```python
from build123d import *

# Parameters (mm, degrees)
SKETCH_1_W          = 30
SKETCH_1_H          = 34
EXTRUDE_1_DEPTH     = 30
HOLE_WIZARD_1_D     = 3.3
HOLE_WIZARD_1_DEPTH = 10
HOLE_WIZARD_2_D     = 3.3
HOLE_WIZARD_2_DEPTH = 10
HOLE_WIZARD_3_D     = 10.5


with BuildPart() as part:
    # 草图1 → 凸台-拉伸1 (new body)
    with BuildSketch(Plane(origin=(0, 0, 0), x_dir=(1, 0, 0), z_dir=(0, 1, 0))):
        with Locations((15, 17)):
            Rectangle(SKETCH_1_W, SKETCH_1_H)
    extrude(amount=EXTRUDE_1_DEPTH)

    # 孔1
    with Locations(Plane(origin=(30, 0, 0), x_dir=(0, 0, -1), z_dir=(1, 0, 0))):
        with Locations((5, 25), (29, 25), (5, 5), (29, 5)):
            Hole(HOLE_WIZARD_1_D / 2, depth=HOLE_WIZARD_1_DEPTH)

    # 孔2
    with Locations(Plane(origin=(0, 30, 0), x_dir=(1, 0, 0), z_dir=(0, 1, 0))):
        with Locations((7, 17), (15, 25), (23, 17), (15, 9)):
            Hole(HOLE_WIZARD_2_D / 2, depth=HOLE_WIZARD_2_DEPTH)

    # 孔3 (through all)
    with Locations(Plane(origin=(0, 30, 0), x_dir=(1, 0, 0), z_dir=(0, 1, 0))):
        with Locations((15, 17)):
            Hole(HOLE_WIZARD_3_D / 2)


solid = part.part
```
Check sheet for the modelled part. Datum: model origin and axes. Units: mm. A direction names the side the tool comes from. Round coordinates to 2 decimals unless told otherwise and drop trailing zeros. Loops run counter-clockwise (first coordinate to the right, second up) from the corner with the lowest first, then second, coordinate; pieces in that order, holes last. Notation, with made-up numbers: (82, 38) -> (89, 38) arc R30 ccw to (89, 61) -> close; hole circle Ø4 at (36.5, -35.75). An arc over 180 degrees is marked (long way). Answer in a Markdown table with one row per item.
Q1. Sectioned sample at A-A on z = -17. Enter the section's corners in (x, y), then the cut area to 3 significant figures.
Data:
| item | result |
|---|---|
| outline | (0, 0) -> (9.75, 0) -> (9.75, 30) -> (8.65, 30) -> (8.65, 20) -> (5.35, 20) -> (5.35, 30) -> (0, 30) -> close; (20.25, 0) -> (30, 0) -> (30, 30) -> (24.65, 30) -> (24.65, 20) -> (21.35, 20) -> (21.35, 30) -> (20.25, 30) -> close |
| area | 519 mm^2 |
Q2. Sectioned sample at C-C on y = 20.75. Enter the section's corners in (x, z).
Data:
| item | result |
|---|---|
| outline | (0, -34) -> (30, -34) -> (30, 0) -> (0, 0) -> close; hole circle Ø3.3 at (7, -17); hole circle Ø10.5 at (15, -17); hole circle Ø3.3 at (15, -25); hole circle Ø3.3 at (15, -9); hole circle Ø3.3 at (23, -17) |
Q3. Sectioned sample at B-B on x = 15. Enter the section's corners in (y, z), then the cut area to 3 significant figures.
Data:
| item | result |
|---|---|
| outline | (0, -34) -> (30, -34) -> (30, -26.65) -> (20, -26.65) -> (20, -23.35) -> (30, -23.35) -> (30, -22.25) -> (0, -22.25) -> close; (0, -11.75) -> (30, -11.75) -> (30, -10.65) -> (20, -10.65) -> (20, -7.35) -> (30, -7.35) -> (30, 0) -> (0, 0) -> close |
| area | 639 mm^2 |
Q4. Sectioned sample at D-D on x = 23. Enter the section's corners in (y, z).
Data:
| item | result |
|---|---|
| outline | (0, -34) -> (30, -34) -> (30, -18.65) -> (20, -18.65) -> (20, -15.35) -> (30, -15.35) -> (30, 0) -> (0, 0) -> close; hole circle Ø3.3 at (5, -29); hole circle Ø3.3 at (5, -5); hole circle Ø3.3 at (25, -29); hole circle Ø3.3 at (25, -5) |
Q5. Release check for a two-part mould opening along X. For faces 4 (the face through (11, 0, -21)), 5 (the face through (8.216, 24.93, -18.115)), 6 (the face through (20, 5, -29)) record: released by +X, released by -X, zero draft, split by the parting line, or undercut.
Data:
| item | result |
|---|---|
| face 4 | zero draft |
| face 5 | undercut |
| face 6 | released by +X |
Q6. Go/stop test with flat-tipped pins: P1, Ø1.6, axis at y = 24.5, z = -29, coming from the +X side; P2, Ø1, axis at x = 15.5, z = -9, coming from the +Y side. Record where each tip stops, or that it passes through.
Data:
| item | result |
|---|---|
| P1 | stops at x = 20 |
| P2 | stops at y = 20 |
Q7. Set-up check for faces 1 (the face through (30, 15, -17)), 2 (the face through (24.93, 4, -6.31)), 3 (the face through (13.476, 24.93, -8.368)): record each of +Z, -Z, +X, -X, +Y, -Y from which the full face is reachable in a straight line by a thin tool's end or side.
Data:
| item | result |
|---|---|
| face 1 | +Z, -Z, +X, +Y, -Y |
| face 2 | +X |
| face 3 | +Y |
Q8. Thickness scan on L1, parallel to Y at x = 22, z = -29; L2, parallel to X at y = 23.5, z = -17; L3, parallel to Z at x = 7, y = 25.25. Record the ranges inside material, lowest first.
Data:
| item | result |
|---|---|
| L1 | y = 0 to 3.35, 6.65 to 23.35, 26.65 to 30 |
| L2 | x = 0 to 5.35, 8.65 to 9.75, 20.25 to 21.35, 24.65 to 30 |
| L3 | z = -34 to -18.65, -15.35 to 0 |
